from build123d import *

# Parameters (mm, degrees)
ARRAY_X_COUNT = 6
ARRAY_X_PITCH = 9
ARRAY_Y_COUNT = 2
ARRAY_Y_PITCH = 8
BOX_W         = 57
BOX_H         = 16
BOX_DEPTH     = 7
FILLET_R      = 0.5


with BuildPart() as array:
    # Cone → Cone (revolve)
    with BuildSketch(Plane(origin=(6, 4, 1), x_dir=(1, 0, 0), z_dir=(0, -1, 0))):
        Polygon((0, 0), (1, 0), (3, 6), (0, 6), align=None)
    revolve(axis=Axis((6, 4, 1), (0, 0, 1)))

    # Array X: Array ×6


with BuildPart() as array_1:
    add(array.part)
    with Locations(*[(i * ARRAY_X_PITCH, 0, 0) for i in range(1, ARRAY_X_COUNT)]):
        add(array.part)

    # Array Y: Array ×2


with BuildPart() as array_2:
    add(array_1.part)
    with Locations(*[(0, i * ARRAY_Y_PITCH, 0) for i in range(1, ARRAY_Y_COUNT)]):
        add(array_1.part)


with BuildPart() as obj1:
    # Box → Box (new body)
    with BuildSketch(Plane.XY):
        with Locations((28.5, 8)):
            Rectangle(BOX_W, BOX_H)
    extrude(amount=BOX_DEPTH)

    # Fillet
    fillet_edges = [obj1.edges().sort_by_distance(p)[0] for p in [
        (0, 0, 3.5),
        (0, 8, 7),
        (0, 16, 3.5),
        (57, 0, 3.5),
        (57, 8, 7),
        (57, 16, 3.5),
        (28.5, 0, 7),
        (28.5, 16, 7),
    ]]
    fillet(fillet_edges, radius=FILLET_R)

    # Cut: cut Array
    add(array_2.part, mode=Mode.SUBTRACT)


solid = obj1.part
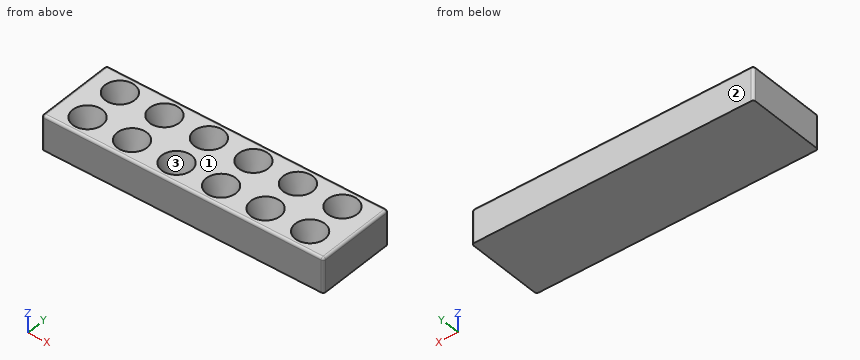
Design review of the part built by this model. Coordinates are the model's own, in mm. Face numbers are marked on the shaded views. Round coordinates to 2 decimals unless told otherwise and drop trailing zeros. Write each loop counter-clockwise with the first axis right and the second up, starting at its lowest first coordinate (ties: lowest second). Pieces come first, ordered by that corner, then holes. Notation, with made-up numbers: (-4, 28) -> (53, 28) arc R29 ccw to (53, 55) -> close; hole circle Ø2 at (23.5, 27). An arc over 180 degrees is marked (long way). One line per question, with ' | ' between items.
(1) Take a section at A-A, the plane z = 3. State how many separate pieces and enclosed holes the cut face has, and give its area (3 significant figures).
Result sheet:
separate pieces: 1 | enclosed holes: 12 | area: 807 mm2
(2) Wall thickness on line 1 (Y direction, x = 7, z = 2); line 2 (Y direction, x = 24, z = 6.75); line 3 (Z direction, x = 26, y = 5.5): over which ranges is each line inside the solid? List them lowest first. Write a range as [from, to].
Result sheet:
line 1: [0, 3.12], [4.88, 11.12], [12.88, 16] | line 2: [0.07, 1.08], [6.92, 9.08], [14.92, 15.93] | line 3: [0, 5.5]
(3) Draft analysis for pull direction Y (two halves, no side actions). For the marked faces 1, 2 and 3, state which applies: released by +Y, released by -Y, zero draft, split by the parting line, or undercut.
Result sheet:
face 1: zero draft | face 2: released by +Y | face 3: undercut
(4) Take a section at B-B, the plane x = 33. State the section outline as (y, z) points, and give its area (3 significant figures).
Result sheet:
outline: (0, 0) -> (16, 0) -> (16, 6.5) arc R0.5 ccw to (15.5, 7) -> (15, 7) -> (13, 1) -> (11, 1) -> (9, 7) -> (7, 7) -> (5, 1) -> (3, 1) -> (1, 7) -> (0.5, 7) arc R0.5 ccw to (0, 6.5) -> close | area: 63.9 mm2
(5) Insertion check: P1, Ø1, axis at x = 42, y = 12, coming from the +Z side. The pin has a flat end and moves straight along its axis. Give the tip position at first contact, or say it passes through.
Result sheet:
P1: z = 1
